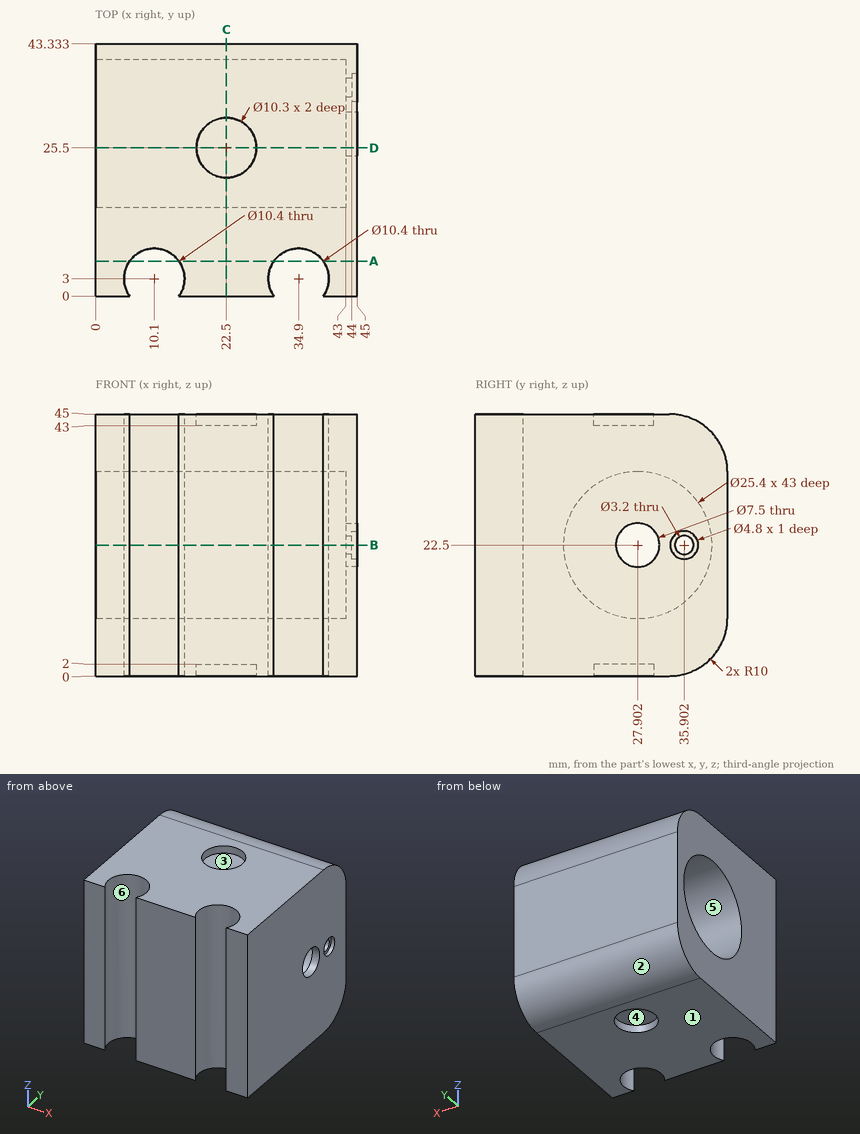
Can you work these out from the drawing? Everything is in mm from the part's minimum corner. A direction names the side the tool comes from. Round coordinates to 2 decimals unless told otherwise and drop trailing zeros. Loops run counter-clockwise (first coordinate to the right, second up) from the corner with the lowest first, then second, coordinate; pieces in that order, holes last. Notation, with made-up numbers: (40.5, 80) - (74.5, 80) arc R31 ccw to (74.5, 110) - close; hole circle Ø10 at (-20, 83). An arc over 180 degrees is marked (long way). Write item = value, one per line. Start each with the question number.
(1) If we section it at B-B (z = 22.5): Please give me the cut outline in (x, y), and give its area (3 significant figures).
(2) If we section it at D-D (y = 25.5): Please give me the cut outline in (x, z).
(3) For the marked faces 4, 5 and 6, which set-ups out of +Z, -Z, +X, -X, +Y, -Y let a thin tool reach every point of the face, with its end or its side?
(4) If I drill on probe 1 along X at (y, z) = (3, 12); probe 2 along Y at (x, z) = (43.8, 22.5); probe 3 along Z at (x, y) = (19, 28.5) (1 decimal), over which ranges is the centre line in solid material (lowest first)? Write a range as [from, to].
(5) If we section it at A-A (y = 6): Please give me the cut outline in (x, z), and give its area (3 significant figures).
(6) If we section it at C-C (x = 22.5): Please give me the cut outline in (y, z).
(7) If we mould it in two halves opening along Y, with no side actions, what happens to the marked faces 1, 2 and 3? For each: released by +Y, released by -Y, zero draft, split by the parting line, or undercut.
(8) For P1, Ø12, axis at x = 22.5, y = 25.5, coming from the -Z side; P2, Ø7.5, axis at y = 35.9, z = 22.5, coming from the -X side; P3, Ø8, axis at x = 22.5, y = 25.5, coming from the +Z side; P4, Ø4, axis at y = 35.9, z = 22.5, coming from the +X side, each with a flat end and sliding along its axis, tell me the tip position at first contact or that it passes through.
Ans:
q1.outline = (0, 0) - (5.85, 0) arc R5.2 cw (long way) to (14.35, 0) - (30.65, 0) arc R5.2 cw (long way) to (39.15, 0) - (45, 0) - (45, 24.15) - (43, 24.15) - (43, 15.2) - (0, 15.2) - close; (0, 40.6) - (43, 40.6) - (43, 37.5) - (44, 37.5) - (44, 38.3) - (45, 38.3) - (45, 43.33) - (0, 43.33) - close; (43, 31.65) - (45, 31.65) - (45, 33.5) - (44, 33.5) - (44, 34.3) - (43, 34.3) - close
q1.area = 691 mm²
q2.outline = (0, 0) - (17.35, 0) - (17.35, 2) - (27.65, 2) - (27.65, 0) - (45, 0) - (45, 19.62) - (43, 19.62) - (43, 10.03) - (0, 10.03) - close; (0, 34.97) - (43, 34.97) - (43, 25.38) - (45, 25.38) - (45, 45) - (27.65, 45) - (27.65, 43) - (17.35, 43) - (17.35, 45) - (0, 45) - close
q3.face_4 = -Z
q3.face_5 = -X
q3.face_6 = +Z, -Z
q4.probe_1 = [0, 4.9], [15.3, 29.7], [40.1, 45]
q4.probe_2 = [0, 24.15], [31.65, 34.3], [37.5, 43.33]
q4.probe_3 = [2, 9.8], [35.2, 43]
q5.outline = (0, 0) - (5.85, 0) - (5.85, 45) - (0, 45) - close; (14.35, 0) - (30.65, 0) - (30.65, 45) - (14.35, 45) - close; (39.15, 0) - (45, 0) - (45, 45) - (39.15, 45) - close
q5.area = 1,260 mm²
q6.outline = (0, 0) - (20.35, 0) - (20.35, 2) - (30.65, 2) - (30.65, 0) - (33.33, 0) arc R10 ccw to (43.33, 10) - (43.33, 35) arc R10 ccw to (33.33, 45) - (30.65, 45) - (30.65, 43) - (20.35, 43) - (20.35, 45) - (0, 45) - close; hole circle Ø25.4 at (27.9, 22.5)
q7.face_1 = zero draft
q7.face_2 = released by +Y
q7.face_3 = undercut
q8.P1 = 0
q8.P2 = 43
q8.P3 = 43
q8.P4 = 44
